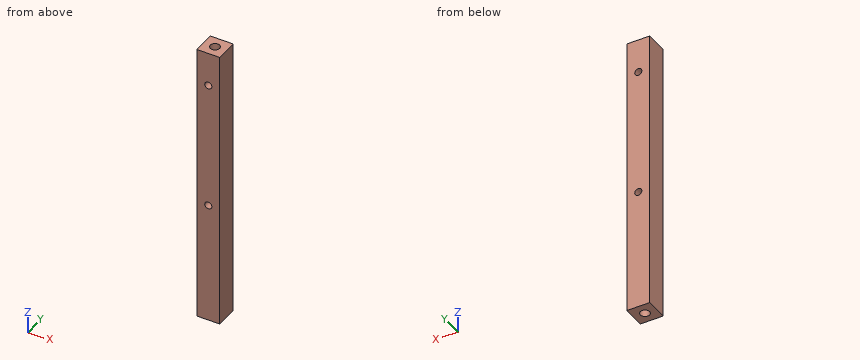
from build123d import *

# Parameters (mm, degrees)
SKETCH1_W                       = 8
SKETCH1_H                       = 8
EXTRUDE1_DEPTH                  = 100
M3_TAPPED_HOLE1_D               = 2.5
M4_TAPPED_HOLE1_D               = 3.3
M4_TAPPED_HOLE1_DEPTH           = 10
M4_TAPPED_HOLE1_TIP             = 0.991420021
M4_TAPPED_HOLE1_ON_FACE_2_D     = 3.3
M4_TAPPED_HOLE1_ON_FACE_2_DEPTH = 10
M4_TAPPED_HOLE1_ON_FACE_2_TIP   = 0.991420021


with BuildPart() as part:
    # Sketch1 → Extrude1 (new body)
    with BuildSketch(Plane.XY):
        with Locations((4, 4)):
            Rectangle(SKETCH1_W, SKETCH1_H)
    extrude(amount=EXTRUDE1_DEPTH)

    # M3 Tapped Hole1 (through all)
    with Locations(Plane(origin=(4, 8, 88), x_dir=(0, 0, 1), z_dir=(0, 1, 0))):
        with Locations((0, 0), (-45, 0)):
            Hole(M3_TAPPED_HOLE1_D / 2)

    # M4 Tapped Hole1
    with Locations(Plane(origin=(4, 4, 100), x_dir=(1, 0, 0), z_dir=(0, 0, 1))):
        with Locations((0, 0)):
            Hole(M4_TAPPED_HOLE1_D / 2, depth=M4_TAPPED_HOLE1_DEPTH)
            with Locations((0, 0, -(M4_TAPPED_HOLE1_DEPTH + M4_TAPPED_HOLE1_TIP / 2))):  # 118° drill point
                Cone(0, M4_TAPPED_HOLE1_D / 2, M4_TAPPED_HOLE1_TIP, mode=Mode.SUBTRACT)

    # M4 Tapped Hole1 on face 2
    with Locations(Plane(origin=(4, 4, 0), x_dir=(-1, 0, 0), z_dir=(0, 0, -1))):
        with Locations((0, 0)):
            Hole(M4_TAPPED_HOLE1_ON_FACE_2_D / 2, depth=M4_TAPPED_HOLE1_ON_FACE_2_DEPTH)
            with Locations((0, 0, -(M4_TAPPED_HOLE1_ON_FACE_2_DEPTH + M4_TAPPED_HOLE1_ON_FACE_2_TIP / 2))):  # 118° drill point
                Cone(0, M4_TAPPED_HOLE1_ON_FACE_2_D / 2, M4_TAPPED_HOLE1_ON_FACE_2_TIP, mode=Mode.SUBTRACT)


solid = part.part
Source: CAD feature listing. Evaluate the final solid. Frame: model axes, mm. Round coordinates to 2 decimals unless told otherwise and drop trailing zeros. Loops run counter-clockwise (first coordinate to the right, second up) from the corner with the lowest first, then second, coordinate; pieces in that order, holes last. Notation, with made-up numbers: (73.5, -26.75) -> (110.5, -26.75) arc R22 cw to (110.5, -2.75) -> close; hole circle Ø2 at (-24.75, 60). An arc over 180 degrees is marked (long way). Answer as a JSON object with one key per item and string values. Group by question number.
Q1. Section query A-A (z = 88). Output: boundary loops of the cut face in (x, y), plus the area to 3 significant figures.
Q2. Contact query for a flat-ended pin moving along its axis: P1, Ø4.5, axis at x = 4, y = 4, coming from the -Z side. Output: stop coordinate, or through.
Q3. Ray query, line 1 (X direction, y = 4, z = 5.5); line 2 (Z direction, x = 5, y = 2.25); line 3 (Z direction, x = 3.25, y = 2.5). Return the intervals inside material, ascending. Write a range as from..to.
Completed:
{
 "1": {"outline": "(0, 0) -> (2.75, 0) -> (2.75, 8) -> (0, 8) -> close; (5.25, 0) -> (8, 0) -> (8, 8) -> (5.25, 8) -> close", "area": "44.0 mm²"},
 "2": {"P1": "z = 0"},
 "3": {"line 1": "0..2.35, 5.65..8", "line 2": "0..42.25, 43.75..87.25, 88.75..100", "line 3": "0..42, 44..87, 89..100"}
}
